Geometry: final body of the model. Coordinates: model frame, mm. Face numbers are marked on the shaded views. A direction names the side the tool comes from. Coordinates: 2 decimals unless noted, no trailing zeros. Order: outer loops, then holes, each group sorted by start corner. A loop starts at its lowest first (then second) coordinate and runs counter-clockwise, first axis right, second up. Notation, with made-up numbers: (66.25, 22) -> (107.25, 22) arc R19 cw to (107.25, 46) -> close; hole circle Ø1 at (80, -15.5). An arc over 180 degrees is marked (long way). Answer in a Markdown table with one row per item. Add a question column.
1) Section query A-A on x = 21.5. Return the cut outline in (y, z).
2) Section query B-B on z = -7.5. Return the cut outline in (x, y).
3) Section query C-C on y = 9. Return the cut outline in (x, z), then the cut area to 3 significant figures.
4) Ray query, line 1 (X direction, y = 4.25, z = -10.1); line 2 (X direction, y = 5.25, z = 27.5); line 3 (X direction, y = 8.5, z = -11). Return the intervals inside material, ascending. Write a range as from..to.
5) Set-up query: the marked faces 1 and 2. Return all of +Z, -Z, +X, -X, +Y, -Y with unobstructed straight access to the full face (end or side cutting, diameter ignored); none if empty.
6) Contact query for flat-ended pins moving along their axis: P1, Ø5, axis at x = -3.5, y = 9, coming from the +Z side; P2, Ø1, axis at x = 1, y = 8.5, coming from the +Z side; P3, Ø6, axis at y = 7.5, z = 2.5, coming from the -X side; P4, Ø13.5, axis at x = 20.5, z = -10.1, coming from the -Y side. Output: stop coordinate, or through.
7) Section query D-D on x = -20.5. Return the cut outline in (y, z), then the cut area to 3 significant figures.
8) Pull-direction query (X, two-part tool) for the marked faces 3, 4, 5 and 6; classes: +X half, -X half, draft (parallel to the pull), parting line (faces both ways), or undercut.
```python
from build123d import *

# Parameters (mm, degrees)
SKETCH1_R           = 7.6
SKETCH1_R_2         = 2.5
BOSS_EXTRUDE1_DEPTH = 10


with BuildPart() as part:
    # Sketch1 → Boss-Extrude1 (new body)
    with BuildSketch(Plane(origin=(0, 0, 0), x_dir=(1, 0, 0), z_dir=(0, 1, 0))):
        with BuildLine():
            Line((-27.5, 25.1), (27.5, 25.1))
            ThreePointArc((27.5, 25.1), (31.035533906, 23.635533906), (32.5, 20.1))
            Line((32.5, 20.1), (32.5, 4.613081447))
            ThreePointArc((32.5, 4.613081447), (31.297772627, 1.360863269), (28.269230769, -0.327392622))
            ThreePointArc((28.269230769, -0.327392622), (11.612250554, -9.612800021), (5, -27.5))
            ThreePointArc((5, -27.5), (0, -32.5), (-5, -27.5))
            ThreePointArc((-5, -27.5), (-11.612250554, -9.612800021), (-28.269230769, -0.327392622))
            ThreePointArc((-28.269230769, -0.327392622), (-31.297772627, 1.360863269), (-32.5, 4.613081447))
            Line((-32.5, 4.613081447), (-32.5, 20.1))
            ThreePointArc((-32.5, 20.1), (-31.035533906, 23.635533906), (-27.5, 25.1))
        make_face()
        with Locations(Location((-20.5, 10.1, 0), (0, 0, 270))):  # turned: the seam where the file's is
            Circle(SKETCH1_R, mode=Mode.SUBTRACT)
        with Locations(Location((20.5, 10.1, 0), (0, 0, 270))):  # turned: the seam where the file's is
            Circle(SKETCH1_R, mode=Mode.SUBTRACT)
        with Locations(Location((0, -27.5, 0), (0, 0, 270))):  # turned: the seam where the file's is
            Circle(SKETCH1_R_2, mode=Mode.SUBTRACT)
        Polygon((7.043673284, 10.1), (3.521836642, 16.2), (-3.521836642, 16.2), (-7.043673284, 10.1), (-3.521836642, 4), (3.521836642, 4), align=None, mode=Mode.SUBTRACT)
    extrude(amount=BOSS_EXTRUDE1_DEPTH)


solid = part.part
```
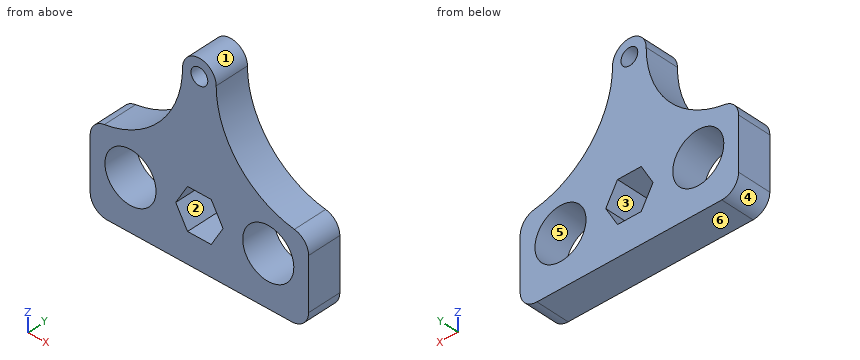
Result:
| question | item | result |
|---|---|---|
| 1 | outline | (0, -25.1) -> (10, -25.1) -> (10, -17.63) -> (0, -17.63) -> close; (0, -2.57) -> (10, -2.57) -> (10, 2.3) -> (0, 2.3) -> close |
| 2 | outline | (-32.5, 0) -> (-27.64, 0) -> (-27.64, 10) -> (-32.5, 10) -> close; (-13.36, 0) -> (-5.54, 0) -> (-5.54, 10) -> (-13.36, 10) -> close; (5.54, 0) -> (13.36, 0) -> (13.36, 10) -> (5.54, 10) -> close; (27.64, 0) -> (32.5, 0) -> (32.5, 10) -> (27.64, 10) -> close |
| 3 | outline | (-32.5, -20.1) arc R5 ccw to (-27.5, -25.1) -> (27.5, -25.1) arc R5 ccw to (32.5, -20.1) -> (32.5, -4.61) arc R5 ccw to (28.27, 0.33) arc R27.5 cw to (5, 27.5) arc R5 ccw to (-5, 27.5) arc R27.5 cw to (-28.27, 0.33) arc R5 ccw to (-32.5, -4.61) -> close; hole circle Ø15.2 at (-20.5, -10.1); hole (-7.04, -10.1) -> (-3.52, -16.2) -> (3.52, -16.2) -> (7.04, -10.1) -> (3.52, -4) -> (-3.52, -4) -> close; hole circle Ø5 at (0, 27.5); hole circle Ø15.2 at (20.5, -10.1) |
| 3 | area | 1,740 mm2 |
| 4 | line 1 | -32.5..-28.1, -12.9..-7.04, 7.04..12.9, 28.1..32.5 |
| 4 | line 2 | -5..-2.5, 2.5..5 |
| 4 | line 3 | -32.5..-28.05, -12.95..-6.52, 6.52..12.95, 28.05..32.5 |
| 5 | face 1 | +Z, +Y, -Y |
| 5 | face 2 | +Y, -Y |
| 6 | P1 | z = 32.4 |
| 6 | P2 | z = 32.47 |
| 6 | P3 | x = -30.34 |
| 6 | P4 | through |
| 7 | outline | (0, -25.1) -> (10, -25.1) -> (10, -17.7) -> (0, -17.7) -> close; (0, -2.5) -> (10, -2.5) -> (10, 2.76) -> (0, 2.76) -> close |
| 7 | area | 127 mm2 |
| 8 | face 3 | undercut |
| 8 | face 4 | -X half |
| 8 | face 5 | undercut |
| 8 | face 6 | draft |
